Read the model definition and answer for the solid it produces. Units are mm, in the model's axes. A direction names the side the tool comes from. Give positions to 0.01 mm unless a question says otherwise; leave off trailing zeros. Write each loop counter-clockwise with the first axis right and the second up, starting at its lowest first coordinate (ties: lowest second). Pieces come first, ordered by that corner, then holes. Notation, with made-up numbers: M 4.25,11.5 L 24.25,11.5 A11 ccw 24.25,21.5 Z; hole C 32.25,-26 d7. An arc over 180 degrees is marked long. Put each result on its own line as item: value.
from build123d import *

# Parameters (mm, degrees)
SKETCH_1_W          = 55
SKETCH_1_H          = 100
EXTRUDE_1_DEPTH     = 1.5
SKETCH_2_R          = 6.1
SKETCH_2_R_2        = 6.5
SKETCH_2_R_3        = 1.6
CUT_EXTRUDE_1_DEPTH = 58.142366069
SKETCH_3_R          = 1.6
CUT_EXTRUDE_2_DEPTH = 58.142366069
SKETCH_4_W          = 30
SKETCH_4_H          = 25
CUT_EXTRUDE_3_DEPTH = 58.142366069
FILLET_1_R          = 5


with BuildPart() as part:
    # ｽｹｯﾁ1 → ﾎﾞｽ - 押し出し1 (new, symmetric)
    with BuildSketch(Plane.XY):
        Rectangle(SKETCH_1_W, SKETCH_1_H)
    extrude(amount=EXTRUDE_1_DEPTH, both=True)

    # ｽｹｯﾁ2 → ｶｯﾄ - 押し出し1 (cut, through all)
    with BuildSketch(Plane.XY.offset(1.5)):
        with Locations((-7.5, 30)):
            Circle(SKETCH_2_R)
        with Locations((-7.5, 0)):
            Circle(SKETCH_2_R_2)
        with Locations((12.923393759, 22.25)):
            Circle(SKETCH_2_R_3)
        with Locations((-0.5, 45.5)):
            Circle(SKETCH_2_R_3)
        with Locations((-13.923393759, 22.25)):
            Circle(SKETCH_2_R_3)
    extrude(amount=-CUT_EXTRUDE_1_DEPTH, mode=Mode.SUBTRACT)

    # ｽｹｯﾁ3 → ｶｯﾄ - 押し出し2 (cut, through all)
    with BuildSketch(Plane.XY.offset(1.5)):
        with Locations((-22.5, 45)):
            Circle(SKETCH_3_R)
        with Locations(Location((22.5, 45, 0), (0, 0, 180))):
            Circle(SKETCH_3_R)
        with Locations((22.5, -45)):
            Circle(SKETCH_3_R)
        with Locations(Location((-22.5, -45, 0), (0, 0, 180))):
            Circle(SKETCH_3_R)
    extrude(amount=-CUT_EXTRUDE_2_DEPTH, mode=Mode.SUBTRACT)

    # ｽｹｯﾁ4 → ｶｯﾄ - 押し出し3 (cut, through all)
    with BuildSketch(Plane.XY.offset(1.5)):
        with Locations((0, -27.5)):
            Rectangle(SKETCH_4_W, SKETCH_4_H)
    extrude(amount=-CUT_EXTRUDE_3_DEPTH, mode=Mode.SUBTRACT)

    # ﾌｨﾚｯﾄ1
    fillet_1_edges = [part.edges().sort_by_distance(p)[0] for p in [
        (15, -15, 0),
        (15, -40, 0),
        (-15, -40, 0),
        (-15, -15, 0),
    ]]
    fillet(fillet_1_edges, radius=FILLET_1_R)


solid = part.part
(1) For a pull along X with two mould halves and no side action, classify faces 3 (the face through (27.5, -1, 0)), 4 (the face through (0, -50, 0)), 5 (the face through (23.24, -46.42, 0.02)) as +X half, -X half, draft (parallel to the pull), parting line (faces both ways), or undercut.
Result:
face 3: +X half
face 4: draft
face 5: undercut
(2) Given pin 1 Ø4 at (x, y) = (-13.92, 22.25) entering from -Z, flat-ended and moving along its own axis, determine where the tip first touches the part or whether it passes through.
Result:
pin 1: stops at z = -1.5
(3) Straight lines are drawn through the part: line 1 along Y through (x, z) = (-7.5, -0.2); line 2 along Y through (x, z) = (22.5, -0.65); line 3 along Y through (x, z) = (10, 0.05). For each, find the intervals that lie inside material, in ascending order. Write a range as from..to.
Result:
line 1: y = -50..-40, -15..-6.5, 6.5..23.9, 36.1..50
line 2: y = -50..-46.6, -43.4..43.4, 46.6..50
line 3: y = -50..-40, -15..50
(4) Section C-C on z = -0.9 is taken. Give the number of separate pieces and of enclosed holes in the cut face, and give its area (3 significant figures).
Result:
separate pieces: 1
enclosed holes: 10
area: 4,470 mm²
(5) Section B-B on x = 22.5 is taken. Determine the outline of the cut face in (y, z).
Result:
outline: M -50,-1.5 L -46.6,-1.5 L -46.6,1.5 L -50,1.5 Z; M -43.4,-1.5 L 43.4,-1.5 L 43.4,1.5 L -43.4,1.5 Z; M 46.6,-1.5 L 50,-1.5 L 50,1.5 L 46.6,1.5 Z
(6) Section A-A on y = 30 is taken. Determine the outline of the cut face in (x, z).
Result:
outline: M -27.5,-1.5 L -13.6,-1.5 L -13.6,1.5 L -27.5,1.5 Z; M -1.4,-1.5 L 27.5,-1.5 L 27.5,1.5 L -1.4,1.5 Z
(7) Which of the six approach directions +Z, -Z, +X, -X, +Y, -Y give full straight-line access (tool end or side, diameter ignored) to faces 1 (the face through (0, -40, 0)), 2 (the face through (0, 50, 0))?
Result:
face 1: +Z, -Z
face 2: +Z, -Z, +X, -X, +Y
(8) Section D-D on y = 0 is taken. Determine the outline of the cut face in (x, z).
Result:
outline: M -27.5,-1.5 L -14,-1.5 L -14,1.5 L -27.5,1.5 Z; M -1,-1.5 L 27.5,-1.5 L 27.5,1.5 L -1,1.5 Z
